Build history of the part. All positions in model axes, mm. A direction names the side the tool comes from. Round coordinates to 2 decimals unless told otherwise and drop trailing zeros. Loops run counter-clockwise (first coordinate to the right, second up) from the corner with the lowest first, then second, coordinate; pieces in that order, holes last. Notation, with made-up numbers: (-26, -16) - (-6, -16) arc R15 cw to (-6, 10) - close; hole circle Ø2 at (-6, 61.5). An arc over 180 degrees is marked (long way). Use one line per item in the form item = value. Start each with the question number.
Q1. Saw through at C-C (z = 4.5). Give the cut face in (x, y).
Q2. Drill centre lines: line 1 (Z direction, x = 15.5, y = 6); line 2 (Y direction, x = 15, z = 5); line 3 (Y direction, x = -8, z = 7.5). Where is each one in solid material? Low to high.
Q3. Pin check, flat tips, straight feed: pin 1 (6.5 mm diameter, centred on x = 4.5, z = -4, fed in from -Y); pin 2 (6.5 mm diameter, centred on x = 24, z = -1.5, fed in from -Y); pin 3 (3 mm diameter, centred on x = 25, y = 33.5, fed in from +Z). Stop position of each tip, or through.
Q4. Saw through at D-D (y = -3.5). Give the cut face in (x, z), then the cut area to 3 significant figures.
Q5. Saw through at B-B (y = 20). Give the cut face in (x, z).
Q6. 3-axis set-ups, long thin cutter, end or side, ignore diameter. For faces 1 (the face through (15.34, 4.06, 14.26)), 2 (the face through (24, 35, 8)), 3 (the face through (3, 41, 0)): which of +Z, -Z, +X, -X, +Y, -Y reach the whole face in a straight line?
Q7. Mould opens along X. For faces 4 (the face through (15.55, 8.62, 15.71)), 5 (the face through (-19, 20, -19)), 6 (the face through (0, 20, -21)) say: released by +X, released by -X, zero draft, split by the parting line, or undercut.
Q8. Saw through at A-A (x = 0). Give the cut face in (y, z), then the cut area to 3 significant figures.
```python
from build123d import *

# Parameters (mm, degrees)
SKETCH1_W                   = 42
SKETCH1_H                   = 42
BOSS_EXTRUDE1_DEPTH         = 41
CHAMFER1_SIZE               = 4
SKETCH2_R                   = 11
BOSS_EXTRUDE2_DEPTH         = 1.7
SKETCH3_R                   = 2.5
BOSS_EXTRUDE3_DEPTH         = 22.5
SKETCH4_W                   = 16
SKETCH4_H                   = 12
BOSS_EXTRUDE4_DEPTH         = 6
TAP_DRILL_FOR_M3_TAP1_D     = 2.5
TAP_DRILL_FOR_M3_TAP1_DEPTH = 8
TAP_DRILL_FOR_M3_TAP1_TIP   = 0.751075774


with BuildPart() as part:
    # Sketch1 → Boss-Extrude1 (new body)
    with BuildSketch(Plane(origin=(0, 0, 0), x_dir=(1, 0, 0), z_dir=(0, 1, 0))):
        Rectangle(SKETCH1_W, SKETCH1_H)
    extrude(amount=BOSS_EXTRUDE1_DEPTH)

    # Chamfer1
    chamfer1_edges = [part.edges().sort_by_distance(p)[0] for p in [
        (21, 20.5, 21),
        (-21, 20.5, 21),
        (-21, 20.5, -21),
        (21, 20.5, -21),
    ]]
    chamfer(chamfer1_edges, length=CHAMFER1_SIZE)

    # Sketch2 → Boss-Extrude2 (add)
    with BuildSketch(Plane(origin=(0, 0, 0), x_dir=(1, 0, 0), z_dir=(0, 1, 0))):
        with Locations(Location((0, 0, 0), (0, 0, 270))):
            Circle(SKETCH2_R)
    extrude(amount=-BOSS_EXTRUDE2_DEPTH)

    # Sketch3 → Boss-Extrude3 (add)
    with BuildSketch(Plane(origin=(0, 0, 0), x_dir=(1, 0, 0), z_dir=(0, 1, 0))):
        with Locations(Location((0, 0, 0), (0, 0, 270))):
            Circle(SKETCH3_R)
    extrude(amount=-BOSS_EXTRUDE3_DEPTH)

    # Sketch4 → Boss-Extrude4 (add)
    with BuildSketch(Plane(origin=(21, 0, 0), x_dir=(0, 0, -1), z_dir=(1, 0, 0))):
        with Locations((0, 35)):
            Rectangle(SKETCH4_W, SKETCH4_H)
    extrude(amount=BOSS_EXTRUDE4_DEPTH)

    # Tap Drill for M3 Tap1
    with Locations(Plane(origin=(0, 0, 0), x_dir=(-1, 0, 0), z_dir=(0, -1, 0))):
        with Locations((-15.5, -15.5), (15.5, -15.5), (15.5, 15.5), (-15.5, 15.5)):
            Hole(TAP_DRILL_FOR_M3_TAP1_D / 2, depth=TAP_DRILL_FOR_M3_TAP1_DEPTH)
            with Locations((0, 0, -(TAP_DRILL_FOR_M3_TAP1_DEPTH + TAP_DRILL_FOR_M3_TAP1_TIP / 2))):  # 118° drill point
                Cone(0, TAP_DRILL_FOR_M3_TAP1_D / 2, TAP_DRILL_FOR_M3_TAP1_TIP, mode=Mode.SUBTRACT)


solid = part.part
```
Report:
q1.outline = (-21, 0) - (-10.04, 0) - (-10.04, -1.7) - (10.04, -1.7) - (10.04, 0) - (21, 0) - (21, 29) - (27, 29) - (27, 41) - (-21, 41) - close
q2.line_1 = -21 to -16.75, -14.25 to 14.25, 16.75 to 21
q2.line_2 = 0 to 41
q2.line_3 = -1.7 to 41
q3.pin_1 = -1.7
q3.pin_2 = 0
q3.pin_3 = 8
q4.outline = circle Ø5 at (0, 0)
q4.area = 19.6 mm²
q5.outline = (-21, -17) - (-17, -21) - (17, -21) - (21, -17) - (21, 17) - (17, 21) - (-17, 21) - (-21, 17) - close
q6.face_1 = -Y
q6.face_2 = +Z, +X, +Y, -Y
q6.face_3 = +Z, -Z, +X, -X, +Y
q7.face_4 = undercut
q7.face_5 = released by -X
q7.face_6 = zero draft
q8.outline = (-22.5, -2.5) - (-1.7, -2.5) - (-1.7, -11) - (0, -11) - (0, -21) - (41, -21) - (41, 21) - (0, 21) - (0, 11) - (-1.7, 11) - (-1.7, 2.5) - (-22.5, 2.5) - close
q8.area = 1,860 mm²
